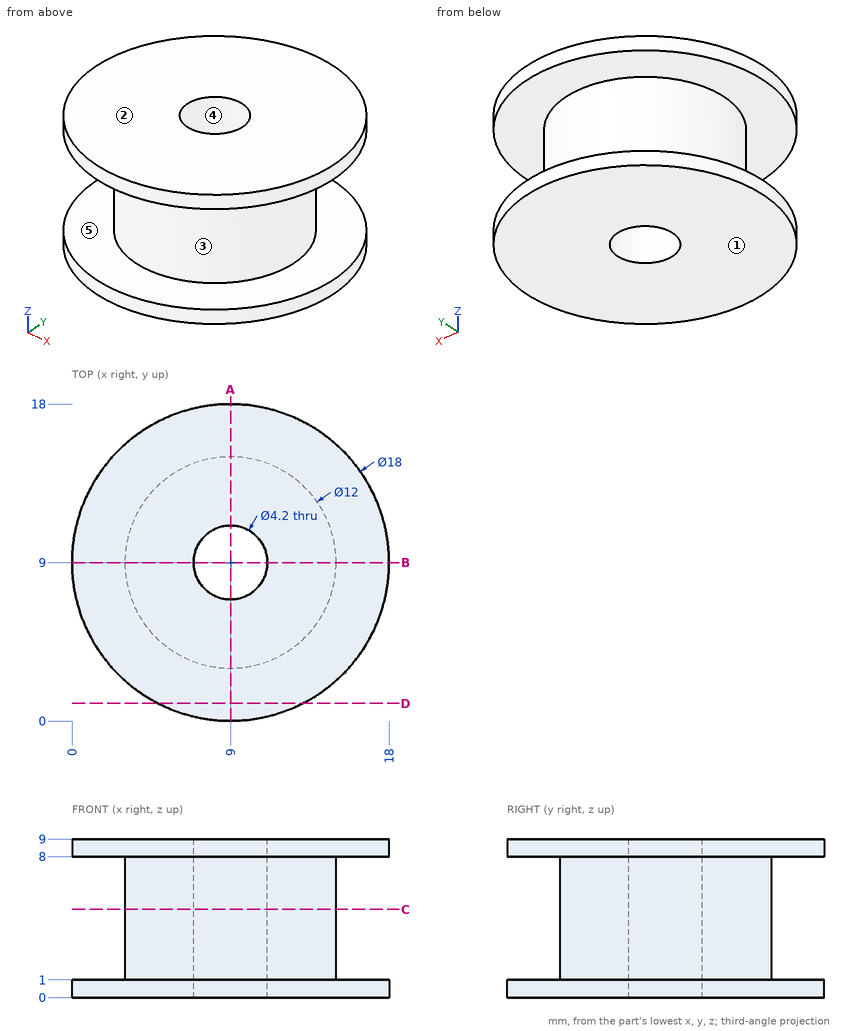
Verification items for this drawing (mm, ordinates from the low corner). A direction names the side the tool comes from. Give positions to 0.01 mm unless a question says otherwise; leave off trailing zeros. Order: outer loops, then holes, each group sorted by start corner. A loop starts at its lowest first (then second) coordinate and runs counter-clockwise, first axis right, second up. Notation, with made-up numbers: M 40.25,-33.75 L 98.25,-33.75 A5 ccw 98.25,-29.75 Z; hole C 88,10.5 d11. An arc over 180 degrees is marked long. Use a Markdown table: item, result.
Item 1: Tool access check on the marked faces 4 and 5. Record the directions out of +Z, -Z, +X, -X, +Y, -Y that give a thin tool (end or side, any length) a straight path to the whole face; none if there is none.
Answers follow:
| item | result |
|---|---|
| face 4 | +Z, -Z |
| face 5 | none |
Item 2: Depth check by flat-ended pin: P1, Ø4, axis at x = 9, y = 9, coming from the +Z side; P2, Ø1.5, axis at y = 8.5, z = 3, coming from the +X side; P3, Ø3, axis at x = 16, z = 3, coming from the +Y side; P4, Ø1.5, axis at x = 5, z = 1, coming from the -Y side. Enter the tip coordinate at first touch or a pass-through.
Answers follow:
| item | result |
|---|---|
| P1 | passes through |
| P2 | stops at x = 15 |
| P3 | stops at y = 11.4 |
| P4 | stops at y = 0.61 |
Item 3: Section check C-C (z = 5). Record the cut outline in (x, y), and give its area (3 significant figures).
Answers follow:
| item | result |
|---|---|
| outline | C 9,9 d12; hole C 9,9 d4.2 |
| area | 99.2 mm2 |
Item 4: Section check A-A (x = 9). Record the cut outline in (y, z), and give its area (3 significant figures).
Answers follow:
| item | result |
|---|---|
| outline | M 0,0 L 6.9,0 L 6.9,9 L 0,9 L 0,8 L 3,8 L 3,1 L 0,1 Z; M 11.1,0 L 18,0 L 18,1 L 15,1 L 15,8 L 18,8 L 18,9 L 11.1,9 Z |
| area | 82.2 mm2 |
Item 5: Draft check along Z on the marked faces 1, 2 and 3. Enter one of: +Z half, -Z half, draft (parallel to the pull), parting line (faces both ways), or undercut.
Answers follow:
| item | result |
|---|---|
| face 1 | -Z half |
| face 2 | +Z half |
| face 3 | undercut |
Item 6: Section check D-D (y = 1). Record the cut outline in (x, z).
Answers follow:
| item | result |
|---|---|
| outline | M 4.88,0 L 13.12,0 L 13.12,1 L 4.88,1 Z; M 4.88,8 L 13.12,8 L 13.12,9 L 4.88,9 Z |
Item 7: Material ranges on line 1 along Z through (x, y) = (14, 14.25); line 2 along Y through (x, z) = (9, 5.25); line 3 along X through (y, z) = (8.5, 4), recorded low to high.
Answers follow:
| item | result |
|---|---|
| line 1 | z = 0 to 1, 8 to 9 |
| line 2 | y = 3 to 6.9, 11.1 to 15 |
| line 3 | x = 3.02 to 6.96, 11.04 to 14.98 |
